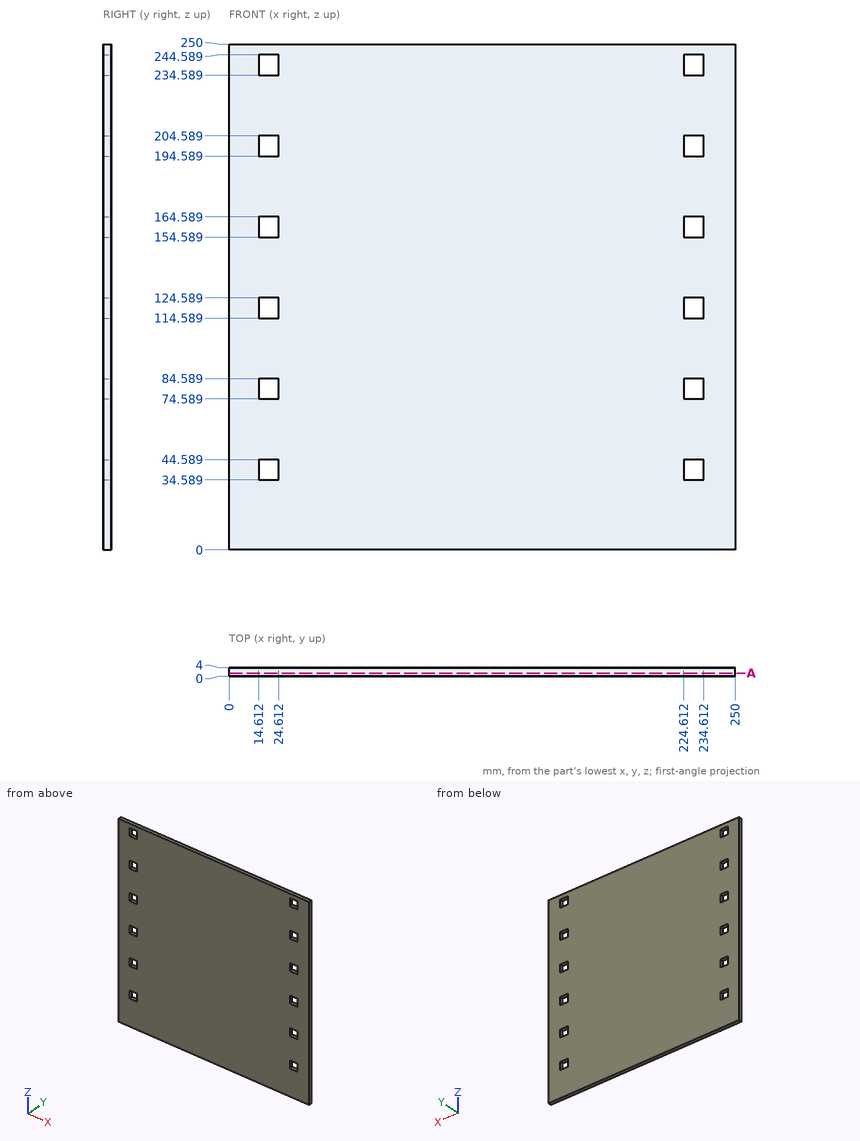
Design review of the part shown in the three views and the two pictorial views. Dimensions are in mm from the part's minimum x, y and z. Round coordinates to 2 decimals unless told otherwise and drop trailing zeros. Answer as CSV lines item,"result". Start each with the question number.
(1) For pin 1 (1.2 mm diameter, centred on x = 21, y = 2, fed in from -Z), flat-tipped, find the tip position at first contact; note if it passes through.
(2) For line 1 (X direction, y = 3, z = 82.5), list the stretches that pass through material, from the lowest coordinate up.
(3) Add section A-A, the plane y = 1.4. State how many separate pieces and enclosed holes the cut face has, plus the area to 3 significant figures.
From the geometry:
1,pin 1,"stops at z = 0"
2,line 1,"x = 0 to 14.61, 24.61 to 224.61, 234.61 to 250"
3,separate pieces,"1"
3,enclosed holes,"12"
3,area,"61,300 mm²"
